Source: three-view drawing plus pictorial views. Frame: mm from the lowest corner of the part. Give positions to 0.01 mm unless a question says otherwise; leave off trailing zeros. Loops run counter-clockwise (first coordinate to the right, second up) from the corner with the lowest first, then second, coordinate; pieces in that order, holes last. Notation, with made-up numbers: M -3.75,39 L 37.25,39 A24 cw 37.25,58 Z; hole C 17.25,-9 d9. An arc over 180 degrees is marked long. One line per item, written item: value. Start each with the question number.
(1) Section B-B on x = 225. Output: boundary loops of the cut face in (y, z), plus the area to 3 significant figures.
(2) Pin query (flat end, axial travel): P1, Ø12, axis at x = 255, y = 75, coming from the +Z side. Return the tip coordinate at first contact, or that it passes through.
(3) Ray query, line 1 along Z through (x, y) = (44, 142.5); line 2 along Y through (x, z) = (225, 167.75); line 3 along Y through (x, z) = (255, 164). Return the intervals inside material, ascending. Write a range as from..to.
(4) Section C-C on y = 75. Output: boundary loops of the cut face in (x, z), plus the area to 3 significant figures.
(5) Section A-A on x = 255. Output: boundary loops of the cut face in (y, z), plus the area to 3 significant figures.
(6) Section D-D on z = 85. Output: boundary loops of the cut face in (x, y).
(7) Pull-direction query (X, two-part tool) for the marked faces 1, 2, 3 and 4; classes: released by +X, released by -X, zero draft, split by the parting line, or undercut.
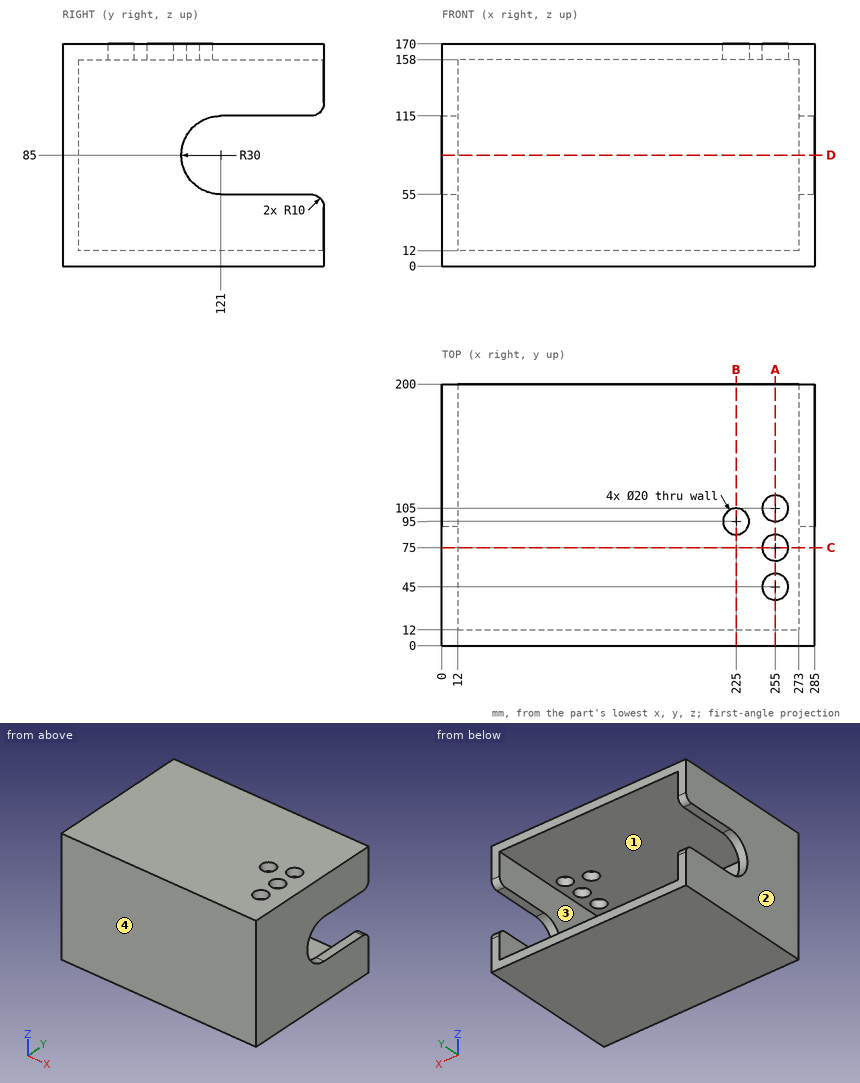
Output values:
1. outline: M 0,0 L 200,0 L 200,12 L 12,12 L 12,158 L 85,158 L 85,170 L 0,170 Z; M 105,158 L 200,158 L 200,170 L 105,170 Z
1. area: 6,310 mm²
2. P1: stops at z = 12
3. line 1: z = 0..12, 158..170
3. line 2: y = 0..85, 105..200
3. line 3: y = 0..35, 55..65, 85..95, 115..200
4. outline: M 0,0 L 285,0 L 285,170 L 265,170 L 265,158 L 273,158 L 273,12 L 12,12 L 12,158 L 245,158 L 245,170 L 0,170 Z
4. area: 10,100 mm²
5. outline: M 0,0 L 200,0 L 200,12 L 12,12 L 12,158 L 35,158 L 35,170 L 0,170 Z; M 55,158 L 65,158 L 65,170 L 55,170 Z; M 85,158 L 95,158 L 95,170 L 85,170 Z; M 115,158 L 200,158 L 200,170 L 115,170 Z
5. area: 5,830 mm²
6. outline: M 0,0 L 285,0 L 285,91 L 273,91 L 273,12 L 12,12 L 12,91 L 0,91 Z
7. face 1: undercut
7. face 2: released by -X
7. face 3: undercut
7. face 4: zero draft
